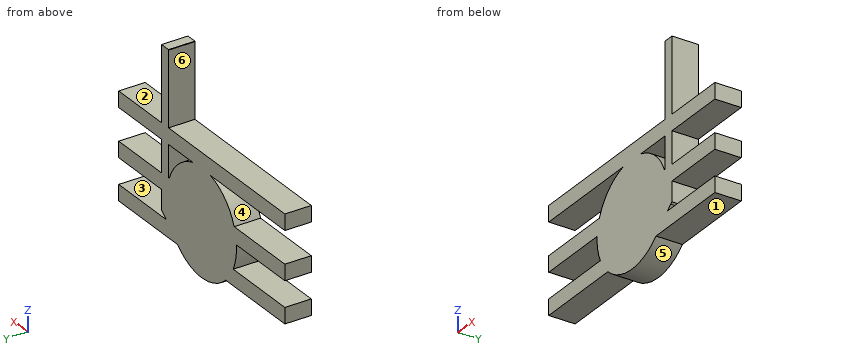
```python
from build123d import *

# Parameters (mm, degrees)
F1_DEPTH = 15
F2_W     = 143
F2_H     = 9
F3_DEPTH = 15
F5_DEPTH = 15


with BuildPart() as f1:
    # F0 (on Front) → F1 (new body)
    with BuildSketch(Plane.XZ):
        with BuildLine():
            ThreePointArc((28.481948, -47.459981), (29.618056, -42.809614), (30, -38.03774))
            ThreePointArc((30, -38.03774), (29.618056, -33.265866), (28.481948, -28.615498))
            ThreePointArc((28.481948, -28.615498), (-29.557796, -32.905813), (23.638915, -56.509385))
            ThreePointArc((23.638915, -56.509385), (26.450312, -52.193338), (28.481948, -47.459981))
        make_face()
        with BuildLine():
            ThreePointArc((28.481948, -28.615498), (29.618056, -33.265866), (30, -38.03774))
            ThreePointArc((30, -38.03774), (29.618056, -42.809614), (28.481948, -47.459981))
            Line((28.481948, -47.459981), (34.471702, -47.459981))
            Line((34.471702, -47.459981), (34.471702, 42.198131))
            Line((34.471702, 42.198131), (28.481948, 42.198131))
            Line((28.481948, 42.198131), (28.481948, -28.615498))
        make_face()
        with BuildLine():
            Line((34.471702, -47.459981), (28.481948, -47.459981))
            ThreePointArc((28.481948, -47.459981), (26.450312, -52.193338), (23.638915, -56.509385))
            Line((23.638915, -56.509385), (34.471702, -47.459981))
        make_face()
    extrude(amount=F1_DEPTH)

    # F2 (on Front) → F3 (join)
    with BuildSketch(Plane.XZ):
        with Locations((-0.117924, -4.5)):
            Rectangle(F2_W, F2_H)
        with Locations((-0.117924, -31.754719)):
            Rectangle(F2_W, F2_H)
        with Locations((-0.117924, -55.231133)):
            Rectangle(F2_W, F2_H)
    extrude(amount=F3_DEPTH)

    # F4 (on Front) → F5 (join)
    with BuildSketch(Plane.XZ):
        with BuildLine():
            ThreePointArc((24.910641, -54.754796), (28.699471, -46.775038), (30, -38.03774))
            ThreePointArc((30, -38.03774), (29.629791, -33.339287), (28.528303, -28.756795))
            ThreePointArc((28.528303, -28.756795), (-29.713704, -33.903032), (24.910641, -54.754796))
        make_face()
        with BuildLine():
            ThreePointArc((28.528303, -28.756795), (29.629791, -33.339287), (30, -38.03774))
            ThreePointArc((30, -38.03774), (28.699471, -46.775038), (24.910641, -54.754796))
            Line((24.910641, -54.754796), (34.471702, -47.547173))
            Line((34.471702, -47.547173), (34.471702, 42.452827))
            Line((34.471702, 42.452827), (28.528303, 42.452827))
            Line((28.528303, 42.452827), (28.528303, -28.756795))
        make_face()
    extrude(amount=F5_DEPTH)


solid = f1.part
```
Input: part model. Units: mm. Frame: model coordinates. Face numbers are marked on the shaded views. A direction names the side the tool comes from. Give positions to 0.01 mm unless a question says otherwise; leave off trailing zeros. Loops run counter-clockwise (first coordinate to the right, second up) from the corner with the lowest first, then second, coordinate; pieces in that order, holes last. Notation, with made-up numbers: M 80.5,82.25 L 100.5,82.25 A25 cw 100.5,94.25 Z; hole C -11,72.5 d4. An arc over 180 degrees is marked long. Answer as CSV lines item,"result". Start each with the question number.
1. Reachability of the marked faces 1, 2 and 3 from +Z, -Z, +X, -X, +Y, -Y: full face, straight path, thin tool, end or side. Return the list, or none.
2. Line query: L1, parallel to Z at x = 40, y = -5; L2, parallel to X at y = -11.25, z = 11; L3, parallel to X at y = -12.5, z = -18. Output: solid intervals per line, ascending.
3. Section B-B on x = 57.5. Return loops of the section in (y, z), plus the area to 3 significant figures.
4. Section C-C on z = -18.5. Return loops of the section in (x, y).
5. Pull-direction query (Z, two-part tool) for the marked faces 4, 5 and 6; classes: released by +Z, released by -Z, zero draft, split by the parting line, or undercut.
6. Pin query (flat end, axial travel): P1, Ø3.5, axis at y = -4.5, z = -43.5, coming from the +X side; P2, Ø2, axis at y = -3, z = -22, coming from the -X side; P3, Ø7.5, axis at x = -25.5, y = -4.5, coming from the -Z side. Return the tip coordinate at first contact, or that it passes through.
7. Section D-D on x = -13.5. Return loops of the section in (y, z), plus the area to 3 significant figures.
Computed values:
1,face 1,"-Z, +X, +Y, -Y"
1,face 2,"+Z, +X, +Y, -Y"
1,face 3,"+X, +Y, -Y"
2,L1,"z = -59.73 to -50.73, -36.25 to -27.25, -9 to 0"
2,L2,"x = 28.48 to 34.47"
2,L3,"x = -22.33 to 22.33, 28.48 to 34.47"
3,outline,"M -15,-59.73 L 0,-59.73 L 0,-50.73 L -15,-50.73 Z; M -15,-36.25 L 0,-36.25 L 0,-27.25 L -15,-27.25 Z; M -15,-9 L 0,-9 L 0,0 L -15,0 Z"
3,area,"405 mm²"
4,outline,"M -22.77,-15 L 22.77,-15 L 22.77,0 L -22.77,0 Z; M 28.48,-15 L 34.47,-15 L 34.47,0 L 28.48,0 Z"
5,face 4,"undercut"
5,face 5,"released by -Z"
5,face 6,"zero draft"
6,P1,"stops at x = 34.47"
6,P2,"stops at x = -25.96"
6,P3,"stops at z = -59.73"
7,outline,"M -15,-64.83 L 0,-64.83 L 0,-11.25 L -15,-11.25 Z; M -15,-9 L 0,-9 L 0,0 L -15,0 Z"
7,area,"939 mm²"
